Source: CAD feature listing. Evaluate the final solid. Frame: model axes, mm. Face numbers are marked on the shaded views. A direction names the side the tool comes from. Round coordinates to 2 decimals unless told otherwise and drop trailing zeros. Loops run counter-clockwise (first coordinate to the right, second up) from the corner with the lowest first, then second, coordinate; pieces in that order, holes last.
(1) Section B-B, the plane y = 0. Return the cut outline in (x, z).
(2) First-contact query: pin 1 Ø2 at (x, z) = (-26.5, -2) entering from -Y; pin 2 Ø3.5 at (x, z) = (-26.5, 0.5) entering from +Y; pin 3 Ø2 at (x, y) = (-11, 2.5) entering from -Z. Flat tips, straight axial feed; report the tip coordinate or a pass-through.
(3) Section D-D, the plane x = -14. Return the cut outline in (y, z), plus the area to 3 significant figures.
(4) Section A-A, the plane z = 0. Return the cut outline in (x, y).
(5) Mould query, pull axis X, two halves, no side actions, for the marked faces 3, 4 and 5. Classes: pulls with the +X half, pulls with the -X half, needs draft (parallel to the pull), parting line crosses it, or undercut.
(6) Section C-C, the plane x = -26. Return the cut outline in (y, z), plus the area to 3 significant figures.
(7) Set-up query: the marked faces 1 and 2. Return all of +Z, -Z, +X, -X, +Y, -Y with unobstructed straight access to the full face (end or side cutting, diameter ignored); none if empty.
(8) Material intervals for probe 1 along X at (y, z) = (-0.9, 0); probe 2 along X at (y, z) = (-3.25, -1); probe 3 along X at (y, z) = (-3.5, -1), sorted ascending.
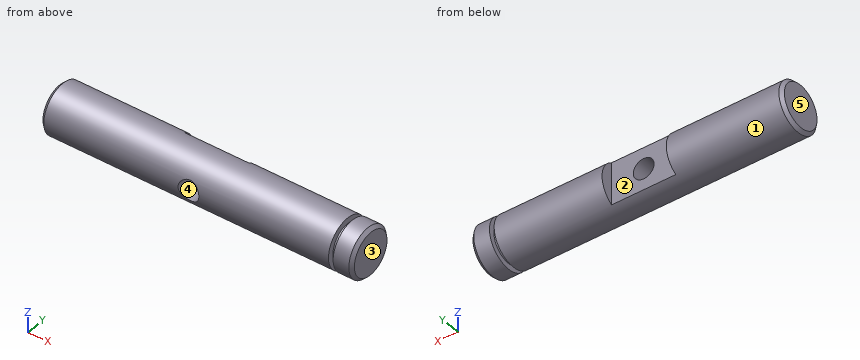
```python
from build123d import *

# Parameters (mm, degrees)
CHAFL_N1_SIZE             = 0.5
CORTAR_EXTRUIR1_DEPTH     = 10.2
TALADRO_ROSCADO_M4X0_71_D = 3.3


with BuildPart() as part:
    # Croquis1 → Revolución1 (revolve)
    with BuildSketch(Plane(origin=(0, 0, 0), x_dir=(0, 1, 0), z_dir=(0, 0, 1)), mode=Mode.PRIVATE) as revoluci_n1_sk:
        Polygon((0, 0), (3.93, 0), (3.93, 3), (3, 3), (3, 3.74), (3.93, 3.74), (3.93, 49.5), (0, 49.5), align=None)
    revolve(revoluci_n1_sk.sketch.rotate(Axis((0, 0, 0), (-1, 0, 0)), 90), axis=Axis((0, 0, 0), (-1, 0, 0)))

    # Chaflán1
    chafl_n1_edges = [part.edges().sort_by_distance(p)[0] for p in [
        (-49.5, 0, 3.93),
        (0, 0, 3.93),
    ]]
    chamfer(chafl_n1_edges, length=CHAFL_N1_SIZE)

    # Croquis2 → Cortar-Extruir1 (cut)
    with BuildSketch(Plane.ZY.offset(31.1)):
        with BuildLine():
            Line((-3.423448554, 1.93), (3.423448554, 1.93))
            ThreePointArc((3.423448554, 1.93), (0, 3.93), (-3.423448554, 1.93))
        make_face()
    extrude(amount=-CORTAR_EXTRUIR1_DEPTH, mode=Mode.SUBTRACT)

    # Taladro roscado M4x0.71 (through all)
    with Locations(Plane(origin=(0, 1.93, 0), x_dir=(-1, 0, 0), z_dir=(0, 1, 0))):
        with Locations((26, 0)):
            Hole(TALADRO_ROSCADO_M4X0_71_D / 2)


solid = part.part
```
Output values:
1. outline: (-49.5, -3.43) - (-49, -3.93) - (-3.74, -3.93) - (-3.74, -3) - (-3, -3) - (-3, -3.93) - (-0.5, -3.93) - (0, -3.43) - (0, 3.43) - (-0.5, 3.93) - (-3, 3.93) - (-3, 3) - (-3.74, 3) - (-3.74, 3.93) - (-49, 3.93) - (-49.5, 3.43) - close; hole circle Ø3.3 at (-26, 0)
2. pin 1: stops at y = -3.74
2. pin 2: stops at y = 1.93
2. pin 3: stops at z = -3.63
3. outline: circle Ø7.86 at (0, 0)
3. area: 48.5 mm2
4. outline: (-49.5, -3.43) - (-49, -3.93) - (-27.65, -3.93) - (-27.65, 1.93) - (-31.1, 1.93) - (-31.1, 3.93) - (-49, 3.93) - (-49.5, 3.43) - close; (-24.35, -3.93) - (-3.74, -3.93) - (-3.74, -3) - (-3, -3) - (-3, -3.93) - (-0.5, -3.93) - (0, -3.43) - (0, 3.43) - (-0.5, 3.93) - (-3, 3.93) - (-3, 3) - (-3.74, 3) - (-3.74, 3.93) - (-20.9, 3.93) - (-20.9, 1.93) - (-24.35, 1.93) - close
5. face 3: pulls with the +X half
5. face 4: undercut
5. face 5: pulls with the -X half
6. outline: (-3.57, -1.65) arc R3.93 ccw to (1.93, -3.42) - (1.93, -1.65) - close; (-3.57, 1.65) - (1.93, 1.65) - (1.93, 3.42) arc R3.93 ccw to start
6. area: 19.9 mm2
7. face 1: +X, -X
7. face 2: +Z, -Z, +Y
8. probe 1: x = -49.5 to -27.65, -24.35 to 0
8. probe 2: x = -49.5 to -27.31, -24.69 to -3.74, -3 to 0
8. probe 3: x = -49.29 to -27.31, -24.69 to -3.74, -3 to -0.21
